Input: part model. Units: mm. Frame: model coordinates. Face numbers are marked on the shaded views. A direction names the side the tool comes from. Round coordinates to 2 decimals unless told otherwise and drop trailing zeros. Loops run counter-clockwise (first coordinate to the right, second up) from the corner with the lowest first, then second, coordinate; pieces in that order, holes last.
1) Section A-A, the plane z = 11. Return loops of the section in (x, y) (3 decimals).
2) Section B-B, the plane y = 102.5. Return loops of the section in (x, z).
3) Access query for the marked faces 4 and 5. Directions: +Z, -Z, +X, -X, +Y, -Y. A direction counts if a zero-diameter tool reaches every point of the face in a straight line with its end or side. Return the directions, or none.
4) First-contact query: pin 1 (1 mm diameter, centred on x = 12.5, y = 62.5, fed in from +Z); pin 2 (2.5 mm diameter, centred on x = 6, y = -101.5, fed in from +Z); pin 3 (1.7 mm diameter, centred on y = -99.5, z = 48, fed in from -X). Flat tips, straight axial feed; report the tip coordinate or a pass-through.
5) Section C-C, the plane y = -58. Return loops of the section in (x, z).
6) Ray query, line 1 along X through (y, z) = (0, 7); line 2 along Z through (x, y) = (2.5, 57.5); line 3 along Y through (x, z) = (-1, 33.5). Return the intervals inside material, ascending.
7) Draft query along Y for the marked faces 1, 2 and 3. Return one class per face: pulls with the +Y half, pulls with the -Y half, needs draft (parallel to the pull), parting line crosses it, or undercut.
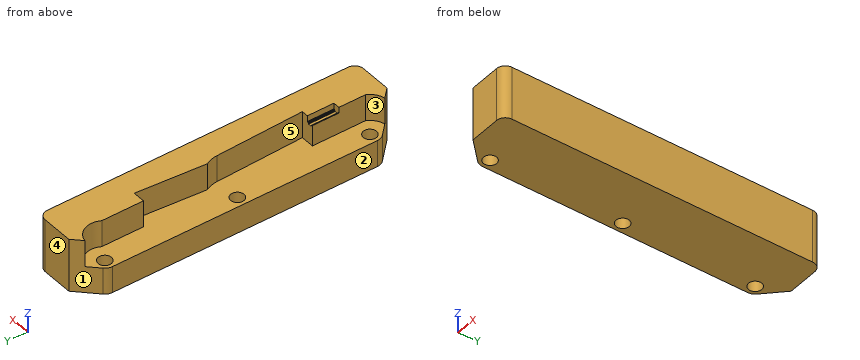
from build123d import *

# Parameters (mm, degrees)
F0_R     = 6.35
F1_DEPTH = 50.8
F2_R     = 8.334375
F4_DEPTH = 25.4
F6_DEPTH = 25.4


with BuildPart() as f1:
    # F0 (on Top) → F1 (new body)
    with BuildSketch(Plane.XY):
        with BuildLine():
            Line((-21.4546158184, 127), (-21.4546158184, -127))
            ThreePointArc((-21.4546158184, -127), (-20.7295683656, -130.6450596933), (-18.6648079092, -133.7351920908))
            Line((-18.6648079092, -133.7351920908), (0, -152.4))
            Line((0, -152.4), (38.1, -152.4))
            Line((38.1, -152.4), (38.1, 152.4))
            Line((38.1, 152.4), (0, 152.4))
            Line((0, 152.4), (-18.6648079092, 133.7351920908))
            ThreePointArc((-18.6648079092, 133.7351920908), (-20.7295683656, 130.6450596933), (-21.4546158184, 127))
        make_face()
        with Locations((-11.9296158184, -127)):
            Circle(F0_R, mode=Mode.SUBTRACT)
        with Locations((-11.9296158184, 0)):
            Circle(F0_R, mode=Mode.SUBTRACT)
        with Locations((-11.9296158184, 127)):
            Circle(F0_R, mode=Mode.SUBTRACT)
    extrude(amount=F1_DEPTH)

    # F2
    f2_edges = [f1.edges().sort_by_distance(p)[0] for p in [
        (38.1, 152.4, 25.4),
        (38.1, -152.4, 25.4),
    ]]
    fillet(f2_edges, radius=F2_R)

    # F3 (on face) → F4 (cut)
    with BuildSketch(Plane.XY.offset(50.8)):
        with BuildLine():
            Line((-18.6648079092, -133.7351920908), (-8.741865195, -143.658134805))
            ThreePointArc((-8.741865195, -143.658134805), (-1.565286118, -140.4251956813), (3.379023496, -134.3007377408))
            Line((3.379023496, -134.3007377408), (3.379023496, -83.5007377408))
            Line((3.379023496, -83.5007377408), (16.079023496, -83.5007377408))
            Line((16.079023496, -83.5007377408), (12.7517639776, 0.9721621486))
            ThreePointArc((12.7517639776, 0.9721621486), (11.7712856877, 6.9557800194), (9.3626122843, 12.5202488115))
            Line((9.3626122843, 12.5202488115), (14.4614139572, 78.7273198366))
            Line((14.4614139572, 78.7273198366), (2.8423227302, 78.7273198366))
            Line((2.8423227302, 78.7273198366), (2.8423227302, 118.6666308892))
            ThreePointArc((2.8423227302, 118.6666308892), (3.4580879019, 134.1325860273), (-8.741865195, 143.658134805))
            Line((-8.741865195, 143.658134805), (-18.6648079092, 133.7351920908))
            ThreePointArc((-18.6648079092, 133.7351920908), (-20.7295683656, 130.6450596933), (-21.4546158184, 127))
            Line((-21.4546158184, 127), (-21.4546158184, -127))
            ThreePointArc((-21.4546158184, -127), (-20.7295683656, -130.6450596933), (-18.6648079092, -133.7351920908))
        make_face()
    extrude(amount=-F4_DEPTH, mode=Mode.SUBTRACT)

    # F5 (on face) → F6 (cut)
    with BuildSketch(Plane(origin=(0, -83.5007377408, 0), x_dir=(-1, 0, 0), z_dir=(0, 1, 0))):
        Polygon((-3.379023496, 50.8), (-9.729023496, 50.8), (-9.729023496, 45.24375), (-8.935273496, 45.24375), (-8.935273496, 44.45), (-8.141523496, 44.45), (-8.141523496, 43.65625), (-4.966523496, 43.65625), (-4.966523496, 44.45), (-4.172773496, 44.45), (-4.172773496, 45.24375), (-3.379023496, 45.24375), align=None)
    extrude(amount=-F6_DEPTH, mode=Mode.SUBTRACT)


solid = f1.part
Final values:
1. outline: (-21.455, -127) arc R9.525 ccw to (-18.665, -133.735) - (0, -152.4) - (29.766, -152.4) arc R8.334 ccw to (38.1, -144.066) - (38.1, 144.066) arc R8.334 ccw to (29.766, 152.4) - (0, 152.4) - (-18.665, 133.735) arc R9.525 ccw to (-21.455, 127) - close; hole circle Ø12.7 at (-11.93, -127); hole circle Ø12.7 at (-11.93, 0); hole circle Ø12.7 at (-11.93, 127)
2. outline: (-21.45, 0) - (38.1, 0) - (38.1, 50.8) - (2.84, 50.8) - (2.84, 25.4) - (-21.45, 25.4) - close
3. face 4: +Z, -Z, +X, -X, +Y
3. face 5: +Z, -X
4. pin 1: stops at z = 25.4
4. pin 2: stops at z = 44.45
4. pin 3: stops at x = 9.73
5. outline: (-21.45, 0) - (38.1, 0) - (38.1, 50.8) - (15.07, 50.8) - (15.07, 25.4) - (-21.45, 25.4) - close
6. line 1: x = -21.45 to -18.28, -5.58 to 38.1
6. line 2: z = 0 to 25.4
6. line 3: y = -151.4 to -139.97, 139.97 to 151.4
7. face 1: pulls with the +Y half
7. face 2: needs draft
7. face 3: undercut
